from build123d import *

# Parameters (mm, degrees)
F0_W     = 140
F0_H     = 100
F1_DEPTH = 2
F2_R     = 30
F3_R     = 3
F4_DEPTH = 25
F5_R     = 5


with BuildPart() as f1:
    # F0 (on Top) → F1 (new body)
    with BuildSketch(Plane.XY):
        Rectangle(F0_W, F0_H)
    extrude(amount=F1_DEPTH)

    # F2
    f2_edges = [f1.edges().sort_by_distance(p)[0] for p in [
        (-70, -50, 1),
        (70, -50, 1),
    ]]
    fillet(f2_edges, radius=F2_R)

    # F3 (on face) → F4 (cut)
    with BuildSketch(Plane.XY.offset(2)):
        with Locations((0, -35)):
            Circle(F3_R)
    extrude(amount=-F4_DEPTH, mode=Mode.SUBTRACT)

    # F5
    f5_edges = [f1.edges().sort_by_distance(p)[0] for p in [
        (70, 50, 1),
        (-70, 50, 1),
    ]]
    fillet(f5_edges, radius=F5_R)


solid = f1.part
The listing builds one solid part. Answer for the finished solid, in the listing's coordinates (mm). Give positions to 0.01 mm unless a question says otherwise; leave off trailing zeros. Loops run counter-clockwise (first coordinate to the right, second up) from the corner with the lowest first, then second, coordinate; pieces in that order, holes last. Notation, with made-up numbers: M 11,49 L 20,49 A20 cw 20,60 Z; hole C -1,-40 d4. An arc over 180 degrees is marked long. Answer as CSV lines item,"result".
Item 1: The part is cut by section A-A (x = 0). Give the vertices of the cut face in (y, z).
Values follow:
outline,"M -50,0 L -38,0 L -38,2 L -50,2 Z; M -32,0 L 50,0 L 50,2 L -32,2 Z"
Item 2: Straight lines are drawn through the part: line 1 along Y through (x, z) = (0, 1.3); line 2 along X through (y, z) = (-25, 0.7); line 3 along Y through (x, z) = (-51, 0.75). For each, find the intervals that lie inside material, in ascending order. Write a range as [from, to].
Values follow:
line 1,"y = [-50, -38], [-32, 50]"
line 2,"x = [-69.58, 69.58]"
line 3,"y = [-47.91, 50]"
Item 3: The part is cut by section C-C (y = -35). Give the vertices of the cut face in (x, z), and give its area (3 significant figures).
Values follow:
outline,"M -65.98,0 L -3,0 L -3,2 L -65.98,2 Z; M 3,0 L 65.98,0 L 65.98,2 L 3,2 Z"
area,"252 mm^2"
Item 4: The part is cut by section B-B (z = 0.8). Give the vertices of the cut face in (x, y).
Values follow:
outline,"M -70,-20 A30 ccw -40,-50 L 40,-50 A30 ccw 70,-20 L 70,45 A5 ccw 65,50 L -65,50 A5 ccw -70,45 Z; hole C 0,-35 d6"
Item 5: The mould has two halves that part along X. Classify faces 1 (the cylindrical face through (-61.445, -40.979, 1.014)), 2 (the cylindrical face through (0, -32, 1)), 3 (the cylindrical face through (68, 49, 1)), 4 (the flat face through (-1, 1, 2)): released by +X, released by -X, zero draft, split by the parting line, or undercut.
Values follow:
face 1,"released by -X"
face 2,"undercut"
face 3,"released by +X"
face 4,"zero draft"
